Check sheet for the modelled part. Datum: model origin and axes. Units: mm. Face numbers are marked on the shaded views. A direction names the side the tool comes from. Give positions to 0.01 mm unless a question says otherwise; leave off trailing zeros. Write each loop counter-clockwise with the first axis right and the second up, starting at its lowest first coordinate (ties: lowest second). Pieces come first, ordered by that corner, then holes. Notation, with made-up numbers: M -25,-0.75 L -10,-0.75 A28 cw -10,25.25 Z; hole C 48.5,54.5 d6. An arc over 180 degrees is marked long. One line per item, written item: value. Start each with the question number.
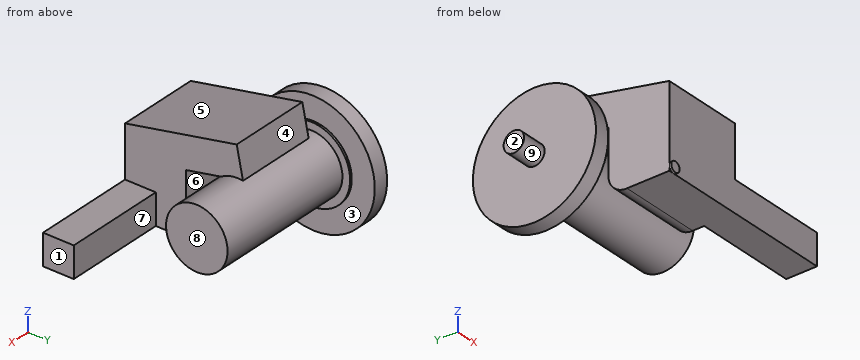
from build123d import *

# Parameters (mm, degrees)
SKETCH1_R           = 76.2
BOSS_EXTRUDE1_DEPTH = 19.05
SKETCH2_R           = 47.625
BOSS_EXTRUDE2_DEPTH = 2.54
SKETCH3_R           = 38.1
BOSS_EXTRUDE3_DEPTH = 177.8
SKETCH4_R           = 12.7
BOSS_EXTRUDE4_DEPTH = 31.75
BOSS_EXTRUDE5_DEPTH = 101.6
SKETCH8_W           = 38.1
SKETCH8_H           = 38.1
BOSS_EXTRUDE6_DEPTH = 127
SKETCH9_R           = 6.35
BOSS_EXTRUDE7_DEPTH = 2.54


with BuildPart() as part:
    # Sketch1 → Boss-Extrude1 (new body)
    with BuildSketch(Plane(origin=(0, 0, 0), x_dir=(0, 0, -1), z_dir=(1, 0, 0))):
        Circle(SKETCH1_R)
    extrude(amount=BOSS_EXTRUDE1_DEPTH)

    # Sketch2 → Boss-Extrude2 (add)
    with BuildSketch(Plane(origin=(19.05, 0, 0), x_dir=(0, 0, -1), z_dir=(1, 0, 0))):
        Circle(SKETCH2_R)
    extrude(amount=BOSS_EXTRUDE2_DEPTH)

    # Sketch3 → Boss-Extrude3 (add)
    with BuildSketch(Plane(origin=(21.59, 0, 0), x_dir=(0, 0, -1), z_dir=(1, 0, 0))):
        Circle(SKETCH3_R)
    extrude(amount=BOSS_EXTRUDE3_DEPTH)

    # Sketch4 → Boss-Extrude4 (add)
    with BuildSketch(Plane.ZY):
        Circle(SKETCH4_R)
    extrude(amount=BOSS_EXTRUDE4_DEPTH)

    # Sketch7 → Boss-Extrude5 (add)
    with BuildSketch(Plane(origin=(34.29, 0, 0), x_dir=(0, 0, -1), z_dir=(1, 0, 0))):
        with BuildLine():
            Line((-37.556058373, 6.415019833), (-75.656058373, -1.41999022))
            Line((-75.656058373, -1.41999022), (-47.219699668, -139.7))
            Line((-47.219699668, -139.7), (54.380300332, -139.7))
            Line((54.380300332, -139.7), (54.380300332, -109.367342085))
            Line((54.380300332, -109.367342085), (54.380300332, -87.28092842))
            ThreePointArc((54.380300332, -87.28092842), (47.900567457, -71.021979596), (31.729146835, -64.326794005))
            Line((31.729146835, -64.326794005), (-23.008477729, -64.326794005))
            Line((-23.008477729, -64.326794005), (-37.556058373, 6.415019833))
        make_face()
    extrude(amount=BOSS_EXTRUDE5_DEPTH)

    # Sketch8 → Boss-Extrude6 (add)
    with BuildSketch(Plane(origin=(135.89, 0, 0), x_dir=(0, 0, -1), z_dir=(1, 0, 0))):
        with Locations((35.330300332, -120.65)):
            Rectangle(SKETCH8_W, SKETCH8_H)
    extrude(amount=BOSS_EXTRUDE6_DEPTH)

    # Sketch9 → Boss-Extrude7 (add)
    with BuildSketch(Plane(origin=(0, -139.7, 0), x_dir=(-1, 0, 0), z_dir=(0, -1, 0))):
        with Locations((-40.64, 48.030300332)):
            Circle(SKETCH9_R)
    extrude(amount=BOSS_EXTRUDE7_DEPTH)


solid = part.part
1) Cross-section at A-A (z = 0). Record the boundary of the cut face in (x, y) (3 decimals), plus the area to 3 significant figures.
2) Material ranges on L1, parallel to X at y = -19.5, z = 44; L2, parallel to X at y = -19.5, z = -18; L3, parallel to Z at x = 240, y = -120.5, recorded low to high. Write a range as from..to.
3) Cross-section at B-B (x = 244.5). Record the boundary of the cut face in (y, z), plus the area to 3 significant figures.
4) Cross-section at D-D (y = 16). Record the boundary of the cut face in (x, z).
5) Tool access check on the marked faces 5, 6, 7, 8 and 9. Record the directions out of +Z, -Z, +X, -X, +Y, -Y that give a thin tool (end or side, any length) a straight path to the whole face; none if there is none.
6) Gauge pin test, flat ends, axial feed: pin 1 (3 mm diameter, centred on y = -30, z = 54, fed in from -X); pin 2 (19 mm diameter, centred on x = 182.5, z = -30, fed in from +Y); pin 3 (8 mm diameter, centred on y = 26.5, z = -34.5, fed in from +X). Record the tip position at first contact, or that the pin passes through.
7) Draft check along X on the marked faces 1, 2, 3 and 4. Enter one of: released by +X, released by -X, zero draft, split by the parting line, or undercut.
8) Cross-section at C-C (z = 43). Record the boundary of the cut face in (x, y).
Data:
1. outline: M -31.75,-12.7 L 0,-12.7 L 0,-76.2 L 19.05,-76.2 L 19.05,-47.625 L 21.59,-47.625 L 21.59,-38.1 L 199.39,-38.1 L 199.39,38.1 L 21.59,38.1 L 21.59,47.625 L 19.05,47.625 L 19.05,76.2 L 0,76.2 L 0,12.7 L -31.75,12.7 Z; M 34.29,-139.7 L 135.89,-139.7 L 135.89,-64.327 L 34.29,-64.327 Z
1. area: 25,200 mm2
2. L1: x = 0..19.05, 34.29..135.89
2. L2: x = 0..199.39
2. L3: z = -54.38..-16.28
3. outline: M -139.7,-54.38 L -101.6,-54.38 L -101.6,-16.28 L -139.7,-16.28 Z
3. area: 1,450 mm2
4. outline: M 0,-74.5 L 19.05,-74.5 L 19.05,-44.86 L 21.59,-44.86 L 21.59,-34.58 L 199.39,-34.58 L 199.39,34.58 L 21.59,34.58 L 21.59,44.86 L 19.05,44.86 L 19.05,74.5 L 0,74.5 Z
5. face 5: +Z, +X, -Y
5. face 6: -Z, +X
5. face 7: +Z, -Z, +X
5. face 8: +Z, -Z, +X, +Y
5. face 9: -X
6. pin 1: stops at x = 0
6. pin 2: stops at y = 32.11
6. pin 3: stops at x = 21.59
7. face 1: released by +X
7. face 2: released by -X
7. face 3: undercut
7. face 4: zero draft
8. outline: M 0,-62.91 L 19.05,-62.91 L 19.05,-20.47 L 21.59,-20.47 L 21.59,20.47 L 19.05,20.47 L 19.05,62.91 L 0,62.91 Z; M 34.29,-139.7 L 135.89,-139.7 L 135.89,5.3 L 34.29,5.3 Z
